from build123d import *

# Parameters (mm, degrees)
SKETCH_2_R          = 317.5
CUT_EXTRUDE_2_DEPTH = 151
CUT_EXTRUDE_3_DEPTH = 772.950427912
SKETCH_4_W          = 192.600523864
SKETCH_4_H          = 200
CUT_EXTRUDE_4_DEPTH = 5


with BuildPart() as part:
    # Эскиз1 → Повернуть1 (revolve)
    with BuildSketch(Plane.XY):
        with BuildLine():
            Line((-671.894470109, 33.485149277), (-10, 150))
            Line((-10, 150), (-9.479899696, 147.045428005))
            Line((-9.479899696, 147.045428005), (-671.374369805, 30.530577282))
            ThreePointArc((-671.374369805, 30.530577282), (-689.74453057, 19.929808529), (-697, 0))
            Line((-697, 0), (-700, 0))
            ThreePointArc((-700, 0), (-692.042388367, 21.858499677), (-671.894470109, 33.485149277))
        make_face()
    revolve(axis=Axis((0, 73.50481492, 0), (0, -1, 0)))

    # Эскиз2 → Вырез-Вытянуть2 (cut, through all)
    with BuildSketch(Plane(origin=(0, 0, 0), x_dir=(1, 0, 0), z_dir=(0, 1, 0))):
        Circle(SKETCH_2_R)
    extrude(amount=CUT_EXTRUDE_2_DEPTH, mode=Mode.SUBTRACT)

    # Эскиз3 → Вырез-Вытянуть3 (cut, through all)
    with BuildSketch(Plane(origin=(-210.975213956, 365.419789709, 0), x_dir=(-0.866025404, -0.5, 0), z_dir=(0.5, -0.866025404, 0))):
        with BuildLine():
            Line((335.939579419, 95.5), (335.939579419, -95.5))
            ThreePointArc((335.939579419, -95.5), (337.111152294, -98.328427125), (339.939579419, -99.5))
            Line((339.939579419, -99.5), (425.439579419, -99.5))
            Line((425.439579419, -99.5), (510.939579419, -99.5))
            ThreePointArc((510.939579419, -99.5), (513.768006544, -98.328427125), (514.939579419, -95.5))
            Line((514.939579419, -95.5), (514.939579419, 95.5))
            ThreePointArc((514.939579419, 95.5), (513.768006544, 98.328427125), (510.939579419, 99.5))
            Line((510.939579419, 99.5), (425.439579419, 99.5))
            Line((425.439579419, 99.5), (339.939579419, 99.5))
            ThreePointArc((339.939579419, 99.5), (337.111152294, 98.328427125), (335.939579419, 95.5))
        make_face()
    extrude(amount=CUT_EXTRUDE_3_DEPTH, mode=Mode.SUBTRACT)

    # Эскиз4 → Вырез-Вытянуть4 (cut)
    with BuildSketch(Plane(origin=(-25.91179023, 147.199009892, 0), x_dir=(0.984857332, 0.173366768, 0), z_dir=(-0.173366768, 0.984857332, 0))):
        with Locations((-506.692199983, 0)):
            Rectangle(SKETCH_4_W, SKETCH_4_H)
    extrude(amount=-CUT_EXTRUDE_4_DEPTH, mode=Mode.SUBTRACT)


solid = part.part
The listing builds one solid part. Answer for the finished solid, in the listing's coordinates (mm). Give positions to 0.01 mm unless a question says otherwise; leave off trailing zeros. Loops run counter-clockwise (first coordinate to the right, second up) from the corner with the lowest first, then second, coordinate; pieces in that order, holes last.
Item 1: A cutting plane is placed at A-A (x = 0). Give the vertices of the cut face in (y, z).
Derived:
outline: (0, -700) arc R34 ccw to (33.49, -671.89) - (95.87, -317.5) - (92.82, -317.5) - (30.53, -671.37) arc R31 cw to (0, -697) - close; (0, 697) arc R31 cw to (30.53, 671.37) - (92.82, 317.5) - (95.87, 317.5) - (33.49, 671.89) arc R34 ccw to (0, 700) - close
Item 2: Each of these flat-tipped pins is pushed along its axis until it touches: pin 1 Ø12 at (x, z) = (79, 384) entering from +Y; pin 2 Ø5 at (y, z) = (15, 2.5) entering from -X; pin 3 Ø12 at (y, z) = (23, -531.5) entering from -X. Where does it stop, or does it pass through?
Derived:
pin 1: stops at y = 83.8
pin 2: stops at x = -697.61
pin 3: stops at x = -451.83
Item 3: Find the intervals of material crossed by line 1 along X through (y, z) = (7.5, 636); line 2 along Y through (x, z) = (-480, -337); line 3 along Y through (x, z) = (-372, -555), in increasing order.
Derived:
line 1: x = -290.4 to -282.9, 282.9 to 290.4
line 2: y = 45.47 to 48.52
line 3: y = 31.1 to 34.15
Item 4: A cutting plane is placed at B-B (z = 0). Give the vertices of the cut face in (x, y).
Derived:
outline: (-700, 0) - (-697, 0) arc R31 cw to (-671.37, 30.53) - (-619.25, 39.71) - (-619.77, 42.66) - (-671.89, 33.49) arc R34 ccw to start; (-430.09, 76.05) - (-429.57, 73.1) - (-317.5, 92.82) - (-317.5, 95.87) - close; (317.5, 92.82) - (671.37, 30.53) arc R31 cw to (697, 0) - (700, 0) arc R34 ccw to (671.89, 33.49) - (317.5, 95.87) - close
Item 5: A cutting plane is placed at C-C (y = 15.5). Give the vertices of the cut face in (x, z).
Derived:
outline: circle Ø1392.52 at (0, 0); hole circle Ø1385.69 at (0, 0)
Item 6: Determine the mould class of faces 1 (the conical face through (43.57, 92.84, -331.86)), 2 (the conical face through (73.627, 88.927, 331.56)) for opening direction X: +X half, -X half, draft (parallel to the pull), parting line (faces both ways), or undercut.
Derived:
face 1: parting line
face 2: undercut
